Can you work these out from the model? Positions are in its coordinate system, mm. Coordinates: 2 decimals unless noted, no trailing zeros. Write each loop counter-clockwise with the first axis right and the second up, starting at its lowest first coordinate (ties: lowest second). Pieces come first, ordered by that corner, then holes. Notation, with made-up numbers: (64, 0) -> (101, 0) arc R23 ccw to (101, 29) -> close; hole circle Ø1 at (17.25, 85.25). An arc over 180 degrees is marked (long way). Use one line per item in the form item = value.
Autodesk Inventor part; units mm, degrees
ref_plane "YZ Plane" through (0, 0, 0) normal (1, 0, 0) x (0, 1, 0)
ref_plane "XZ Plane" through (0, 0, 0) normal (0, 1, 0) x (-1, 0, 0)
ref_plane "XY Plane" through (0, 0, 0) normal (0, 0, 1) x (1, 0, 0)
sketch "スケッチ1" plane through (0, 0, 0) normal (0, 1, 0) x (-1, 0, 0)
  line L0 (0, 0) -> (97.5, 0)
  line L1 (97.5, 0) -> (97.5, -60)
  line L2 (97.5, -60) -> (0, -60)
  line L3 (0, -60) -> (0, 0)
  dimension "d0" = 97.5
  dimension "d1" = 60
extrude "押し出し1" add sketch "スケッチ1" along normal blind 3
sketch "スケッチ2" plane through (0, 3, 0) normal (0, 1, 0) x (1, 0, 0)
  line L0 (0, 0) -> (0, 60)
  line L1 (-97.5, 0) -> (0, 0)
  line L2 (-97.5, 60) -> (-97.5, 0)
  point P0 (-15, 30)
  point P1 (-15, 10)
  point P2 (-15, 50)
  point P3 (-82.5, 30)
  point P4 (-82.5, 10)
  point P5 (-82.5, 50)
  dimension "d4" = 15
  dimension "d5" = 30
  dimension "d6" = 20
  dimension "d7" = 20
  dimension "d8" = 15
  dimension "d9" = 15
  dimension "d10" = 15
  dimension "d11" = 15
  dimension "d12" = 15
  dimension "d13" = 20
  dimension "d14" = 20
  dimension "d15" = 30
hole "穴1" at (-15, 3, -30) at (-15, 3, -10) at (-15, 3, -50) at (-82.5, 3, -30) at (-82.5, 3, -10) at (-82.5, 3, -50) direction (0, -1, 0) diameter 3.2 end through all
fillet "フィレット1" radius 6 4 edges at (-97.5, 1.5, 0) (0, 1.5, 0) (-97.5, 1.5, -60) (0, 1.5, -60)
properties part number "足回り_固定"
Q1. Will this pin go through, and if not, where does the flat tip stop? pin 1 (8 mm diameter, centred on x = -79.5, z = -50.5, fed in from -Y).
Return value:
pin_1 = 0
Q2. Suppose I cut it at A-A (x = -15). Write out the boundary of the cut face in (y, z), then the cut area to 3 significant figures.
Return value:
outline = (0, -60) -> (3, -60) -> (3, -51.6) -> (0, -51.6) -> close; (0, -48.4) -> (3, -48.4) -> (3, -31.6) -> (0, -31.6) -> close; (0, -28.4) -> (3, -28.4) -> (3, -11.6) -> (0, -11.6) -> close; (0, -8.4) -> (3, -8.4) -> (3, 0) -> (0, 0) -> close
area = 151 mm2
Q3. Suppose I cut it at B-B (z = -50). Write out the boundary of the cut face in (x, y), then the cut area to 3 significant figures.
Return value:
outline = (-97.5, 0) -> (-84.1, 0) -> (-84.1, 3) -> (-97.5, 3) -> close; (-80.9, 0) -> (-16.6, 0) -> (-16.6, 3) -> (-80.9, 3) -> close; (-13.4, 0) -> (0, 0) -> (0, 3) -> (-13.4, 3) -> close
area = 273 mm2
Q4. If I drill on line 1 (Z direction, x = -82.5, y = 2.45); line 2 (X direction, y = 2, z = -50); line 3 (Z direction, x = -81.5, y = 1.65), over which ranges is the centre line in solid material (lowest first)? Write a range as from..to.
Return value:
line_1 = -60..-51.6, -48.4..-31.6, -28.4..-11.6, -8.4..0
line_2 = -97.5..-84.1, -80.9..-16.6, -13.4..0
line_3 = -60..-51.25, -48.75..-31.25, -28.75..-11.25, -8.75..0
Q5. Thinking about a two-plate mould opening in X: for faces 1 (the flat face through (-48, 0, -30)), 2 (the cylindrical face through (-16.08, 1.48, -31.18)), 3 (the cylindrical face through (-15.07, 1.48, -11.6)), 4 (the cylindrical face through (-1.804, 1.521, -1.711)), which applies, released by +X, released by -X, zero draft, split by the parting line, or undercut?
Return value:
face_1 = zero draft
face_2 = undercut
face_3 = undercut
face_4 = released by +X
